Autodesk Inventor part; units mm, degrees
ref_plane "YZ Plane" through (0, 0, 0) normal (1, 0, 0) x (0, 1, 0)
ref_plane "XZ Plane" through (0, 0, 0) normal (0, 1, 0) x (-1, 0, 0)
ref_plane "XY Plane" through (0, 0, 0) normal (0, 0, 1) x (1, 0, 0)
sketch "Sketch1" plane through (0, 0, 0) normal (1, 0, 0) x (0, 1, 0)
  line L0 (0, 0) -> (8.128, 0)
  line L1 (8.128, 0) -> (8.128, -12.7)
  line L2 (0, -12.7) -> (0, 0)
  arc A0 (8.128, -12.7) -> (0, -12.7) centre (4.064, -17.8157) ccw
  line L3 (8.128, 0) -> (6.0753, 0)
  line L4 (4.064, 0) -> (4.064, -17.8157) construction
  dimension "d1" = 8.128
  dimension "d2" = 12.7
revolve "Revolution1" add sketch "Sketch1" angle 360 about axis through (0, 8.128, 0) along (0, -1, 0)
sketch "Sketch2" plane through (0, 0, 0) normal (0, -1, 0) x (1, 0, 0)
  circle A0 centre (0, 0) radius 5.5
  dimension "d3" = 11
extrude "Extrusion1" cut sketch "Sketch2" against normal blind 1.4
sketch "Sketch3" plane through (0, 1.4, 0) normal (0, -1, 0) x (1, 0, 0)
  circle A0 centre (0, 0) radius 3.925
  dimension "d6" = 7.85
extrude "Extrusion2" cut sketch "Sketch3" against normal through all
properties part number "top - top pullet"
Check sheet for the modelled part. Datum: model origin and axes. Units: mm. A direction names the side the tool comes from. Give positions to 0.01 mm unless a question says otherwise; leave off trailing zeros. Order: outer loops, then holes, each group sorted by start corner. A loop starts at its lowest first (then second) coordinate and runs counter-clockwise, first axis right, second up. Notation, with made-up numbers: (78.5, 76.5) -> (96.5, 76.5) arc R29 cw to (96.5, 104.5) -> close; hole circle Ø8 at (-2, 89.5). An arc over 180 degrees is marked (long way). Use CSV: the item, a comma, the result in double quotes. Start each with the question number.
1) Go/stop test with flat-tipped pins: P1, Ø3, axis at x = 4.5, y = 4, coming from the -Z side; P2, Ø1, axis at x = -4.5, y = 4, coming from the -Z side; P3, Ø6.5, axis at x = 0, z = 0, coming from the -Y side; P4, Ø2, axis at y = 6, z = -1, coming from the -X side. Record where each tip stops, or that it passes through.
2) Mould release check, pull along X, two halves, no side actions. Record for faces 1 (the face through (-3, 0, -5)), 2 (the face through (-1, 1.4, 4)): released by +X, released by -X, zero draft, split by the parting line, or undercut.
3) Set-up check for faces 3 (the face through (-2.893, 4.717, 2.653)), 4 (the face through (-1.19, 0.69, -5.37)): record each of +Z, -Z, +X, -X, +Y, -Y from which the full face is reachable in a straight line by a thin tool's end or side.
4) Sectioned sample at D-D, the plane y = 7.25. Record the boundary of the cut face in (x, z) (3 decimals).
5) Sectioned sample at A-A, the plane x = 0. Record the boundary of the cut face in (y, z) (3 decimals).
6) Sectioned sample at C-C, the plane y = 3. Record the boundary of the cut face in (x, z) (3 decimals).
7) Sectioned sample at B-B, the plane z = 0. Record the boundary of the cut face in (x, y) (3 decimals).
8) Material ranges on line 1 (Z direction, x = 0, y = 6.75) (3 decimals); line 2 (Z direction, x = 0, y = 6) (3 decimals); line 3 (Y direction, x = 4.5, z = -11.25), recorded low to high. Write a range as from..to.
Recorded:
1,P1,"z = -10.88"
1,P2,"z = -10.55"
1,P3,"through"
1,P4,"x = -11.94"
2,face 1,"zero draft"
2,face 2,"undercut"
3,face 3,"+Y, -Y"
3,face 4,"-Y"
4,outline,"circle Ø24.223 at (0, 0); hole circle Ø7.85 at (0, 0)"
5,outline,"(0, -12.7) arc R6.533 cw to (8.128, -12.7) -> (8.128, -3.925) -> (1.4, -3.925) -> (1.4, -5.5) -> (0, -5.5) -> close; (0, 5.5) -> (1.4, 5.5) -> (1.4, 3.925) -> (8.128, 3.925) -> (8.128, 12.7) arc R6.533 cw to (0, 12.7) -> close"
6,outline,"circle Ø22.739 at (0, 0); hole circle Ø7.85 at (0, 0)"
7,outline,"(-12.7, 0) -> (-5.5, 0) -> (-5.5, 1.4) -> (-3.925, 1.4) -> (-3.925, 8.128) -> (-12.7, 8.128) arc R6.533 cw to start; (3.925, 1.4) -> (5.5, 1.4) -> (5.5, 0) -> (12.7, 0) arc R6.533 cw to (12.7, 8.128) -> (3.925, 8.128) -> close"
8,line 1,"-11.86..-3.925, 3.925..11.86"
8,line 2,"-11.576..-3.925, 3.925..11.576"
8,line 3,"0..0.87, 7.26..8.13"
